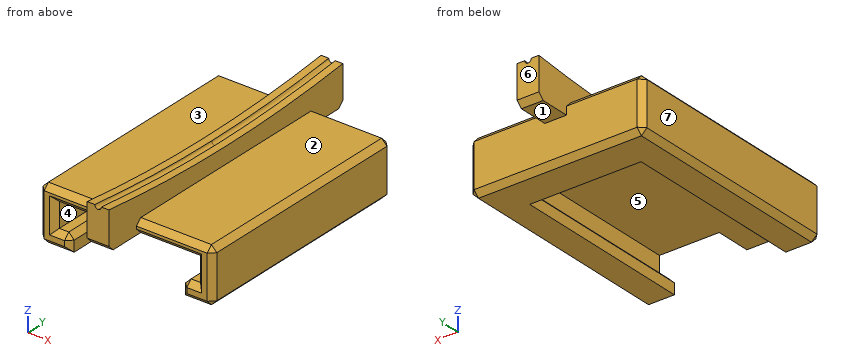
from build123d import *

# Parameters (mm, degrees)
BOX001_W        = 20.5
BOX001_H        = 35
BOX001_DEPTH    = 3
BOX002_W        = 26
BOX002_H        = 37
BOX002_DEPTH    = 4.5
BOX_W           = 32
BOX_H           = 42
BOX_DEPTH       = 10
CHAMFER001_SIZE = 1
CYLINDER_R      = 241
CYLINDER_DEPTH  = 10
TORUS_R         = 0.6
BOX003_W        = 4
BOX003_H        = 55
BOX003_DEPTH    = 20
CHAMFER_SIZE    = 1


with BuildPart() as clamp_mount_hole:
    # Box001 → Box001 (new body)
    with BuildSketch(Plane(origin=(4.75, 0, 0), x_dir=(1, 0, 0), z_dir=(0, 0, 1))):
        with Locations((10.25, 17.5)):
            Rectangle(BOX001_W, BOX001_H)
    extrude(amount=BOX001_DEPTH)


with BuildPart() as clamp_mount_shape:
    # Box002 → Box002 (new body)
    with BuildSketch(Plane(origin=(2, 0, 3), x_dir=(1, 0, 0), z_dir=(0, 0, 1))):
        with Locations((13, 18.5)):
            Rectangle(BOX002_W, BOX002_H)
    extrude(amount=BOX002_DEPTH)

    # Fusion: union clamp_mount_hole
    add(clamp_mount_hole.part)


with BuildPart() as obj1:
    # Box → Box (new body)
    with BuildSketch(Plane(origin=(-1, 0, 0), x_dir=(1, 0, 0), z_dir=(0, 0, 1))):
        with Locations((16, 21)):
            Rectangle(BOX_W, BOX_H)
    extrude(amount=BOX_DEPTH)

    # Cut: cut clamp_mount_shape
    add(clamp_mount_shape.part, mode=Mode.SUBTRACT)

    # Chamfer001
    chamfer001_edges = [obj1.edges().sort_by_distance(p)[0] for p in [
        (-1, 0, 5),
        (-1, 21, 10),
        (-1, 42, 5),
        (-1, 21, 0),
        (1.875, 0, 0),
        (4.75, 0, 1.5),
        (3.375, 0, 3),
        (2, 0, 5.25),
        (15, 0, 7.5),
        (28, 0, 5.25),
        (26.625, 0, 3),
        (25.25, 0, 1.5),
        (28.125, 0, 0),
        (31, 0, 5),
        (15, 0, 10),
        (15, 42, 10),
        (31, 21, 10),
        (15, 42, 0),
        (31, 42, 5),
        (31, 21, 0),
        (4.75, 17.5, 3),
        (25.25, 17.5, 3),
        (15, 35, 3),
    ]]
    chamfer(chamfer001_edges, length=CHAMFER001_SIZE)


with BuildPart() as cylinder:
    # Cylinder → Cylinder (new body)
    with BuildSketch(Plane(origin=(10, 0, 0), x_dir=(0, 0, -1), z_dir=(1, 0, 0))):
        Circle(CYLINDER_R)
    extrude(amount=CYLINDER_DEPTH)


with BuildPart() as cut_disk:
    # Torus → Torus (revolve)
    with BuildSketch(Plane(origin=(15, 0, 0), x_dir=(0, 0, -1), z_dir=(0, -1, 0))):
        with Locations((241, 0)):
            Circle(TORUS_R)
    revolve(axis=Axis((15, 0, 0), (1, 0, 0)))

    # Fusion001: union Cylinder
    add(cylinder.part)


with BuildPart() as cut_disk_1:
    # Fusion001 placement: moved
    add(cut_disk.part.moved(Location((0, 21, 254))))


with BuildPart() as fret_wire_clamp:
    # Box003 → Box003 (new body)
    with BuildSketch(Plane(origin=(13, -6.5, 7.5), x_dir=(1, 0, 0), z_dir=(0, 0, 1))):
        with Locations((2, 27.5)):
            Rectangle(BOX003_W, BOX003_H)
    extrude(amount=BOX003_DEPTH)

    # Cut001: cut cut_disk
    add(cut_disk_1.part, mode=Mode.SUBTRACT)

    # Chamfer
    chamfer_edges = [fret_wire_clamp.edges().sort_by_distance(p)[0] for p in [
        (15, -6.5, 7.5),
        (15, 48.5, 7.5),
    ]]
    chamfer(chamfer_edges, length=CHAMFER_SIZE)

    # Fusion002: union obj1
    add(obj1.part)


solid = fret_wire_clamp.part
Check sheet for the modelled part. Datum: model origin and axes. Units: mm. Face numbers are marked on the shaded views. A direction names the side the tool comes from. Coordinates: 2 decimals unless noted, no trailing zeros. Write each loop counter-clockwise with the first axis right and the second up, starting at its lowest first coordinate (ties: lowest second). Pieces come first, ordered by that corner, then holes. Notation, with made-up numbers: M 65,4 L 104,4 A17 ccw 104,36 Z; hole C -38.75,24.5 d4. An arc over 180 degrees is marked long. Answer as CSV lines item,"result".
Q1. Set-up check for the marked faces 1, 2 and 3: record each of +Z, -Z, +X, -X, +Y, -Y from which the full face is reachable in a straight line by a thin tool's end or side.
Check result:
face 1,"-Z, +X, -X, +Y"
face 2,"+Z, +X, +Y, -Y"
face 3,"+Z, -X, +Y, -Y"
Q2. Go/stop test with flat-tipped pins: pin 1 (2.5 mm diameter, centred on x = 20.5, z = 5.5, fed in from -Y); pin 2 (1 mm diameter, centred on x = 3.5, y = 16, fed in from +Z); pin 3 (3 mm diameter, centred on x = 8, y = 13.5, fed in from -Z). Record where each tip stops, or that it passes through.
Check result:
pin 1,"y = 37"
pin 2,"z = 10"
pin 3,"z = 7.5"
Q3. Material ranges on probe 1 along X at (y, z) = (6.5, 3.5); probe 2 along Z at (x, y) = (27.5, 18); probe 3 along Y at (x, z) = (21.5, 7), recorded low to high. Write a range as from..to.
Check result:
probe 1,"-1..2, 28..31"
probe 2,"0..3, 7.5..10"
probe 3,"37..42"
Q4. Cross-section at B-B (x = 8.5). Record the boundary of the cut face in (y, z), then the cut area to 3 significant figures.
Check result:
outline,"M 0,8.5 L 1,7.5 L 37,7.5 L 37,3 L 36,3 L 35,2 L 35,0 L 41,0 L 42,1 L 42,9 L 41,10 L 1,10 L 0,9 Z"
area,"146 mm^2"
Q5. Cross-section at C-C (x = 27). Record the boundary of the cut face in (y, z), then the cut area to 4 significant figures.
Check result:
outline,"M 0,1 L 1,0 L 41,0 L 42,1 L 42,9 L 41,10 L 1,10 L 0,9 L 0,8.5 L 1,7.5 L 37,7.5 L 37,3 L 1,3 L 0,2 Z"
area,"250.5 mm^2"
Q6. Cross-section at A-A (z = 6.25). Record the boundary of the cut face in (x, y), then the cut area to 3 significant figures.
Check result:
outline,"M -1,1 L 0,0 L 1,0 L 2,1 L 2,37 L 28,37 L 28,1 L 29,0 L 30,0 L 31,1 L 31,41 L 30,42 L 0,42 L -1,41 Z"
area,"379 mm^2"
Q7. Mould release check, pull along X, two halves, no side actions. Record for the marked faces 4, 5, 6 and 7: released by +X, released by -X, zero draft, split by the parting line, or undercut.
Check result:
face 4,"undercut"
face 5,"undercut"
face 6,"zero draft"
face 7,"released by -X"
